```python
from build123d import *

# Parameters (mm, degrees)
F0_R      = 19.05
F0_R_2    = 2.15265
F1_DEPTH  = 10.922
F5_DEPTH  = 6.477
F7_DEPTH  = 6.477
F8_R      = 11.1125
F8_R_2    = 2.15265
F9_DEPTH  = 14.478
F10_R     = 6.35
F10_R_2   = 2.15265
F11_DEPTH = 7.9375
F12_R     = 2.15265
F13_DEPTH = 3.175
F14_R     = 0.762
F15_SIZE  = 3.175


with BuildPart() as f1:
    # F0 (on Top) → F1 (new body)
    with BuildSketch(Plane.XY):
        Circle(F0_R)
        with Locations((-7.540625, -13.060746)):
            Circle(F0_R_2, mode=Mode.SUBTRACT)
        with Locations((7.540625, -13.060746)):
            Circle(F0_R_2, mode=Mode.SUBTRACT)
        with Locations((-15.08125, 0)):
            Circle(F0_R_2, mode=Mode.SUBTRACT)
        with Locations((-7.540625, 13.060746)):
            Circle(F0_R_2, mode=Mode.SUBTRACT)
        Circle(F0_R_2, mode=Mode.SUBTRACT)
        with Locations((15.08125, 0)):
            Circle(F0_R_2, mode=Mode.SUBTRACT)
        with Locations((7.540625, 13.060746)):
            Circle(F0_R_2, mode=Mode.SUBTRACT)
    extrude(amount=F1_DEPTH)

    # F4 (on face) → F5 (cut, through all)
    with BuildSketch(Plane.XY.offset(10.922)):
        with BuildLine():
            Line((-6.087962, 18.482159), (-12.962038, 14.513409))
            Line((-12.962038, 14.513409), (-10.977663, 11.076371))
            ThreePointArc((-10.977663, 11.076371), (-5.55625, 9.623707), (-4.103587, 15.045121))
            Line((-4.103587, 15.045121), (-6.087962, 18.482159))
        make_face()
        with BuildLine():
            Line((19.05, 3.96875), (15.08125, 3.96875))
            ThreePointArc((15.08125, 3.96875), (11.1125, 0), (15.08125, -3.96875))
            Line((15.08125, -3.96875), (19.05, -3.96875))
            Line((19.05, -3.96875), (19.05, 3.96875))
        make_face()
        with BuildLine():
            Line((-10.977663, -11.076371), (-12.962038, -14.513409))
            Line((-12.962038, -14.513409), (-6.087962, -18.482159))
            Line((-6.087962, -18.482159), (-4.103587, -15.045121))
            ThreePointArc((-4.103587, -15.045121), (-5.55625, -9.623707), (-10.977663, -11.076371))
        make_face()
    extrude(amount=-F5_DEPTH, mode=Mode.SUBTRACT)

    # F6 (on face) → F7 (cut, through all)
    with BuildSketch(Plane(origin=(0, 0, 0), x_dir=(1, 0, 0), z_dir=(0, 0, -1))):
        with BuildLine():
            Line((4.103587, -15.045121), (6.087962, -18.482159))
            Line((6.087962, -18.482159), (12.962038, -14.513409))
            Line((12.962038, -14.513409), (10.977663, -11.076371))
            ThreePointArc((10.977663, -11.076371), (5.55625, -9.623707), (4.103587, -15.045121))
        make_face()
        with BuildLine():
            Line((12.962038, 14.513409), (6.087962, 18.482159))
            Line((6.087962, 18.482159), (4.103587, 15.045121))
            ThreePointArc((4.103587, 15.045121), (5.55625, 9.623707), (10.977663, 11.076371))
            Line((10.977663, 11.076371), (12.962038, 14.513409))
        make_face()
        with BuildLine():
            Line((-15.08125, 3.96875), (-19.05, 3.96875))
            Line((-19.05, 3.96875), (-19.05, -3.96875))
            Line((-19.05, -3.96875), (-15.08125, -3.96875))
            ThreePointArc((-15.08125, -3.96875), (-11.1125, 0), (-15.08125, 3.96875))
        make_face()
    extrude(amount=-F7_DEPTH, mode=Mode.SUBTRACT)

    # F8 (on face) → F9 (join)
    with BuildSketch(Plane.XY.offset(10.922)):
        Circle(F8_R)
        Circle(F8_R_2, mode=Mode.SUBTRACT)
    extrude(amount=F9_DEPTH)

    # F10 (on face) → F11 (join)
    with BuildSketch(Plane.XY.offset(25.4)):
        Circle(F10_R)
        Circle(F10_R_2, mode=Mode.SUBTRACT)
    extrude(amount=F11_DEPTH)

    # F12 (on face) → F13 (join)
    with BuildSketch(Plane.XY.offset(33.3375)):
        Polygon((3.175, 5.499261), (-3.175, 5.499261), (-6.35, 0), (-3.175, -5.499261), (3.175, -5.499261), (6.35, 0), align=None)
        Circle(F12_R, mode=Mode.SUBTRACT)
    extrude(amount=F13_DEPTH)

    # F14
    f14_edges = [f1.edges().sort_by_distance(p)[0] for p in [
        (-12.75304, -14.151413, 7.6835),
        (5.878963, -18.120163, 3.2385),
        (12.75304, -14.151413, 3.2385),
        (18.632003, 3.96875, 7.6835),
        (18.632003, -3.96875, 7.6835),
        (-5.878963, -18.120163, 7.6835),
        (12.75304, 14.151413, 3.2385),
        (5.878963, 18.120163, 3.2385),
        (-5.878963, 18.120163, 7.6835),
        (-12.75304, 14.151413, 7.6835),
        (-18.632003, 3.96875, 3.2385),
        (-18.632003, -3.96875, 3.2385),
    ]]
    fillet(f14_edges, radius=F14_R)

    # F15
    f15_edges = [f1.edges().sort_by_distance(p)[0] for p in [
        (-11.1125, 0, 25.4),
    ]]
    chamfer(f15_edges, length=F15_SIZE)


solid = f1.part
```
Geometry: final body of the model. Coordinates: model frame, mm. A direction names the side the tool comes from. Give positions to 0.01 mm unless a question says otherwise; leave off trailing zeros. Loops run counter-clockwise (first coordinate to the right, second up) from the corner with the lowest first, then second, coordinate; pieces in that order, holes last. Notation, with made-up numbers: (31.5, 77.5) -> (82.5, 77.5) arc R15 cw to (82.5, 85.5) -> close; hole circle Ø1 at (16, 12.5). An arc over 180 degrees is marked (long way). Return JSON: item names as keys, results as strings.
Item 1: Line query: line 1 (Z direction, x = 10.5, y = 12); line 2 (Y direction, x = 0, z = 8.5); line 3 (Z direction, x = -4.5, y = -16.5). Output: solid intervals per line, ascending.
Filled in:
{"line 1": "6.48 to 10.92", "line 2": "-19.05 to -2.15, 2.15 to 19.05", "line 3": "0 to 10.92"}
Item 2: Section B-B, the plane z = 34.5. Output: boundary loops of the cut face in (x, y) (3 decimals), plus the area to 3 significant figures.
Filled in:
{"outline": "(-6.35, 0) -> (-3.175, -5.499) -> (3.175, -5.499) -> (6.35, 0) -> (3.175, 5.499) -> (-3.175, 5.499) -> close; hole circle Ø4.305 at (0, 0)", "area": "90.2 mm^2"}
Item 3: Section C-C, the plane y = 12.5. Output: boundary loops of the cut face in (x, z) (3 decimals), plus the area to 3 significant figures.
Filled in:
{"outline": "(-14.375, 0) -> (-9.619, 0) -> (-9.619, 4.445) -> (-11.8, 4.445) -> (-11.8, 10.922) -> (-14.375, 10.922) -> close; (-5.462, 0) -> (3.612, 0) -> (3.612, 6.477) -> (5.462, 6.477) -> (5.462, 10.922) -> (-3.612, 10.922) -> (-3.612, 4.445) -> (-5.462, 4.445) -> close; (9.619, 6.477) -> (11.8, 6.477) -> (11.8, 0) -> (14.375, 0) -> (14.375, 10.922) -> (9.619, 10.922) -> close", "area": "171 mm^2"}
Item 4: Mould query, pull axis X, two halves, no side actions, for faces 5 (the flat face through (-12, 0, 10.922)), 6 (the cylindrical face through (5.6, 9.6, 3.2)), 7 (the flat face through (7, 16, 6.477)), 8 (the flat face through (-4.76, -16.18, 7.73)). Classes: released by +X, released by -X, zero draft, split by the parting line, or undercut.
Filled in:
{"face 5": "zero draft", "face 6": "undercut", "face 7": "undercut", "face 8": "released by -X"}
Item 5: Pin query (flat end, axial travel): P1, Ø1.3, axis at x = -16.5, z = 3, coming from the +Y side; P2, Ø10, axis at y = -6, z = 30, coming from the +X side; P3, Ø12, axis at x = -3.5, z = 27.5, coming from the +Y side. Return the tip coordinate at first contact, or that it passes through.
Filled in:
{"P1": "y = 10.57", "P2": "x = 6.83", "P3": "y = 11.09"}
Item 6: Section D-D, the plane z = 3.5. Output: boundary loops of the cut face in (x, y), plus the area to 3 significant figures.
Filled in:
{"outline": "(-18.4, -4.93) arc R19.05 ccw to (4.93, -18.4) arc R0.76 ccw to (5.4, -17.28) -> (4.1, -15.05) arc R3.97 cw to (10.98, -11.08) -> (12.27, -13.31) arc R0.76 ccw to (13.47, -13.47) arc R19.05 ccw to (13.47, 13.47) arc R0.76 ccw to (12.27, 13.31) -> (10.98, 11.08) arc R3.97 cw to (4.1, 15.05) -> (5.4, 17.28) arc R0.76 ccw to (4.93, 18.4) arc R19.05 ccw to (-18.4, 4.93) arc R0.76 ccw to (-17.67, 3.97) -> (-15.08, 3.97) arc R3.97 cw to (-15.08, -3.97) -> (-17.67, -3.97) arc R0.76 ccw to start; hole circle Ø4.31 at (-7.54, -13.06); hole circle Ø4.31 at (-7.54, 13.06); hole circle Ø4.31 at (0, 0); hole circle Ø4.31 at (15.08, 0)", "area": "915 mm^2"}
Item 7: Access query for faces 1 (the flat face through (5, 3, 33.338)), 2 (the flat face through (0, -5.499, 35)), 3 (the cylindrical face through (11.113, 0.087, 7.729)), 4 (the flat face through (11.63, 12.21, 3.19)). Directions: +Z, -Z, +X, -X, +Y, -Y. A direction counts if a zero-diameter tool reaches every point of the face in a straight line with its end or side. Return the directions, or none.
Filled in:
{"face 1": "+Z, +X, +Y", "face 2": "+Z, +X, -X, -Y", "face 3": "+Z, +X", "face 4": "-Z, +Y"}
